Autodesk Inventor part; units mm, degrees
ref_plane "YZ Plane" through (0, 0, 0) normal (1, 0, 0) x (0, 1, 0)
ref_plane "XZ Plane" through (0, 0, 0) normal (0, 1, 0) x (-1, 0, 0)
ref_plane "XY Plane" through (0, 0, 0) normal (0, 0, 1) x (1, 0, 0)
sketch "Sketch1" plane through (0, 0, 0) normal (0, 1, 0) x (-1, 0, 0)
  line L0 (0, 0) -> (25.4, 0)
  line L1 (25.4, 0) -> (25.4, 50.8)
  line L2 (25.4, 50.8) -> (0, 50.8)
  line L3 (0, 50.8) -> (0, 0)
  line L4 (22.86, 48.26) -> (2.54, 48.26)
  line L5 (2.54, 48.26) -> (2.54, 2.54)
  line L6 (2.54, 2.54) -> (22.86, 2.54)
  line L7 (22.86, 2.54) -> (22.86, 48.26)
  dimension "d0" = 50.8
  dimension "d1" = 25.4
  dimension "d2" = 2.54
  dimension "d3" = 2.54
  dimension "d4" = 2.54
  dimension "d5" = 2.54
extrude "Extrusion1" add sketch "Sketch1" along normal blind 762
sketch "Sketch2" plane through (0, 0, 50.8) normal (1, 0, 0) x (0, 0, -1)
  line L0 (0, 0) -> (50.8, 0)
  line L1 (0, 0) -> (0, 762)
  line L2 (50.8, 0) -> (0, 0)
  line L3 (0, 0) -> (0, 25.4)
  line L4 (0, 25.4) -> (50.8, 25.4)
  line L5 (50.8, 25.4) -> (50.8, 0)
  line L6 (48.26, 0) -> (48.26, 762)
  line L7 (2.54, 0) -> (2.54, 762)
  line L8 (48.26, 2.54) -> (2.54, 2.54)
  line L9 (2.54, 2.54) -> (2.54, 22.86)
  line L10 (2.54, 22.86) -> (48.26, 22.86)
  line L11 (48.26, 22.86) -> (48.26, 2.54)
  dimension "d8" = 25.4
  dimension "d9" = 2.54
  dimension "d10" = 2.54
extrude "Extrusion2" add sketch "Sketch2" along normal blind 406.4 contours L1 L4 L7 L0 | L7 L8 L6 L0 | L6 L4 L5 L0 | L4 L6 L10 L7
sketch "Sketch3" plane through (-25.4, 762, 50.8) normal (0, 0, 1) x (1, 0, 0)
  point P0 (25.4, -762)
sketch "Sketch4" plane through (0, 0, 0) normal (0, -1, 0) x (1, 0, 0)
  line L0 (0, 0) -> (406.4, 0)
  line L1 (406.4, 0) -> (431.8, 0)
  line L2 (431.8, 0) -> (431.8, 50.8)
  line L3 (431.8, 50.8) -> (406.4, 50.8)
  line L4 (406.4, 50.8) -> (406.4, 0)
  line L5 (408.94, 48.26) -> (429.26, 48.26)
  line L6 (429.26, 48.26) -> (429.26, 2.54)
  line L7 (429.26, 2.54) -> (408.94, 2.54)
  line L8 (408.94, 2.54) -> (408.94, 48.26)
  dimension "d13" = 25.4
  dimension "d14" = 2.54
  dimension "d15" = 2.54
  dimension "d16" = 2.54
  dimension "d17" = 2.54
extrude "Extrusion3" add sketch "Sketch4" against normal blind 762
sketch "Sketch6" plane through (-25.4, 0, 0) normal (0, 0, -1) x (-1, 0, 0)
  circle A0 centre (-12.7, 12.7) radius 2.5797
  line L0 (0, 0) -> (0, 762)
  line L1 (-457.2, 0) -> (0, 0)
  circle A1 centre (-12.7, 38.1) radius 2.5797
  circle A2 centre (-12.7, 63.5) radius 2.5797
  circle A3 centre (-38.1, 13.2387) radius 2.5797
  circle A4 centre (-63.5, 12.7) radius 2.5797
  circle A5 centre (-12.7, 12.7) radius 2.5797
  line L2 (0, 0) -> (0, 762)
  line L3 (-457.2, 0) -> (0, 0)
  circle A6 centre (-12.7, 38.1) radius 2.5797
  circle A7 centre (-12.7, 63.5) radius 2.5797
  circle A8 centre (-38.1, 13.2387) radius 2.5797
  circle A9 centre (-63.5, 12.7) radius 2.5797
  line L4 (-25.4, 2.54) -> (-431.8, 2.54)
  line L5 (-228.6, 2.54) -> (-228.6, 762)
  circle A10 centre (-444.5, 12.7) radius 2.5797
  circle A11 centre (-444.5, 38.1) radius 2.5797
  circle A12 centre (-419.1, 13.2387) radius 2.5797
  circle A13 centre (-393.7, 12.7) radius 2.5797
  circle A14 centre (-444.5, 63.5) radius 2.5797
  point P0 (-25.4, 0)
  point P1 (-25.4, 0)
  dimension "d22" = 12.7
  dimension "d23" = 12.7
  dimension "d24" = 5.1594
  dimension "d25" = 25.4
  dimension "d26" = 5.1594
  dimension "d27" = 25.4
  dimension "d28" = 5.1594
  dimension "d29" = 25.4
  dimension "d30" = 5.1594
  dimension "d31" = 12.7
  dimension "d32" = 5.1594
  dimension "d33" = 25.4
  dimension "d36" = 12.7
  dimension "d37" = 12.7
  dimension "d38" = 5.1594
  dimension "d39" = 25.4
  dimension "d40" = 5.1594
  dimension "d41" = 25.4
  dimension "d42" = 5.1594
  dimension "d43" = 25.4
  dimension "d44" = 5.1594
  dimension "d45" = 12.7
  dimension "d46" = 5.1594
  dimension "d47" = 25.4
extrude "Extrusion6" cut sketch "Sketch6" against normal blind 736.6
sketch "Sketch8" plane through (-25.4, 0, 50.8) normal (0, 0, 1) x (1, 0, 0)
  line L0 (25.4, 25.4) -> (25.4, 762)
  line L1 (0, 0) -> (25.4, 0)
  line L2 (25.4, 0) -> (25.4, 25.4)
  line L3 (25.4, 25.4) -> (0, 25.4)
  line L4 (0, 25.4) -> (0, 0)
  line L5 (2.54, 2.54) -> (22.86, 2.54)
  line L6 (22.86, 2.54) -> (22.86, 22.86)
  line L7 (22.86, 22.86) -> (2.54, 22.86)
  line L8 (2.54, 22.86) -> (2.54, 2.54)
  line L9 (0, 0) -> (457.2, 0)
  point P0 (25.4, 0)
  dimension "d50" = 25.4
  dimension "d51" = 2.54
  dimension "d52" = 0
  dimension "d53" = 2.54
  dimension "d54" = 2.54
  dimension "d55" = 2.54
extrude "Extrusion7" add sketch "Sketch8" along normal blind 127
sketch "Sketch10" plane through (406.4, 762, 50.8) normal (0, 0, 1) x (1, 0, 0)
  line L0 (0, -736.6) -> (0, 0)
  line L1 (0, -736.6) -> (0, -762)
  point P0 (-406.4, -762)
sketch "Sketch11" plane through (406.4, 762, 50.8) normal (0, 0, 1) x (1, 0, 0)
  line L0 (-406.4, -762) -> (-406.4, -736.6)
  line L1 (-406.4, -762) -> (-406.4, -736.6)
sketch "Sketch12" plane through (406.4, 762, 50.8) normal (0, 0, 1) x (1, 0, 0)
  line L0 (0, -736.6) -> (0, 0)
  line L1 (25.4, -762) -> (25.4, 0)
  line L2 (0, -736.6) -> (25.4, -736.6)
  line L3 (25.4, -736.6) -> (25.4, -762)
  line L4 (25.4, -762) -> (0, -762)
  line L5 (0, -762) -> (0, -736.6)
  line L6 (22.86, -762) -> (22.86, 0)
  line L7 (22.86, -739.14) -> (2.54, -739.14)
  line L8 (2.54, -739.14) -> (2.54, -759.46)
  line L9 (2.54, -759.46) -> (22.86, -759.46)
  line L10 (22.86, -759.46) -> (22.86, -739.14)
  point P0 (-406.4, -762)
  dimension "d62" = 2.54
  dimension "d63" = 2.54
  dimension "d64" = 2.54
extrude "Extrusion9" add sketch "Sketch12" along normal blind 127 contours L4 L6 L2 L1 | L4 L5 L2 L6 L7 L8 L9
sketch "Sketch9" plane through (-25.4, 0, 0) normal (-1, 0, 0) x (0, 0, 1)
  circle A0 centre (64.7925, 12.7) radius 9.525
  line L0 (0, 0) -> (177.8, 0)
  dimension "d58" = 19.05
  dimension "d59" = 12.7
extrude "Extrusion8" cut sketch "Sketch9" against normal blind 508
sketch "Sketch13" plane through (0, 0, 50.8) normal (1, 0, 0) x (0, 0, -1)
  line L0 (-127, 0) -> (-101.6, 0)
  line L1 (-101.6, 0) -> (-101.6, 25.4)
  line L2 (-101.6, 25.4) -> (-127, 25.4)
  line L3 (-127, 25.4) -> (-127, 0)
  line L4 (0, 0) -> (-127, 0)
  line L5 (-127, 0) -> (-127, 25.4)
  line L6 (0, 2.54) -> (-127, 2.54)
  line L7 (-104.14, 2.54) -> (-124.46, 2.54)
  line L8 (-124.46, 2.54) -> (-124.46, 22.86)
  line L9 (-124.46, 22.86) -> (-104.14, 22.86)
  line L10 (-104.14, 22.86) -> (-104.14, 2.54)
  point P0 (50.8, 0)
  dimension "d67" = 25.4
  dimension "d68" = 25.4
  dimension "d69" = 0
  dimension "d70" = 0
  dimension "d71" = 2.54
  dimension "d72" = 2.54
  dimension "d73" = 2.54
extrude "Extrusion10" add sketch "Sketch13" along normal blind 406.4 contours L3 L6 L1 L0 | L3 L2 L1 L6 L10 L9 L8
sketch "Sketch14" plane through (-25.4, 25.4, 50.8) normal (0, 1, 0) x (1, 0, 0)
  line L0 (457.2, -127) -> (0, -127)
  line L1 (228.6, -127) -> (228.6, 50.8)
  line L2 (25.4, 50.8) -> (431.8, 50.8)
  circle A0 centre (444.5, -114.3) radius 2.5797
  circle A1 centre (419.1, -114.3) radius 2.5797
  circle A2 centre (393.7, -114.3) radius 2.5797
  circle A3 centre (444.5, -88.9) radius 2.5797
  circle A4 centre (444.5, -63.5) radius 2.5797
  line L3 (457.2, 0) -> (457.2, -127)
  circle A5 centre (12.7, -114.3) radius 2.5797
  circle A6 centre (38.1, -114.3) radius 2.5797
  circle A7 centre (63.5, -114.3) radius 2.5797
  circle A8 centre (12.7, -88.9) radius 2.5797
  circle A9 centre (12.7, -63.5) radius 2.5797
  dimension "d76" = 90
  dimension "d77" = 228.6
  dimension "d78" = 12.7
  dimension "d79" = 12.7
  dimension "d80" = 12.7
  dimension "d81" = 12.7
  dimension "d82" = 12.7
  dimension "d83" = 12.7
  dimension "d84" = 5.1594
  dimension "d85" = 5.1594
  dimension "d86" = 5.1594
  dimension "d87" = 5.1594
  dimension "d88" = 5.1594
  dimension "d89" = 25.4
  dimension "d90" = 25.4
  dimension "d91" = 25.4
  dimension "d92" = 25.4
extrude "Extrusion11" cut sketch "Sketch14" against normal blind 406.4
properties part number "battery shelf frame"
Could you check a few things on this model? Use its own coordinates, in mm. A direction names the side the tool comes from. Give positions to 0.01 mm unless a question says otherwise; leave off trailing zeros. Order: outer loops, then holes, each group sorted by start corner. A loop starts at its lowest first (then second) coordinate and runs counter-clockwise, first axis right, second up. Notation, with made-up numbers: (60, 26.5) -> (76, 26.5) arc R35 ccw to (76, 65.5) -> close; hole circle Ø1 at (23, 63.25). An arc over 180 degrees is marked (long way). Answer in a Markdown table with one row per item. Add a question column.
Item 1: We'd pull the mould along Y, two halves only. Please class faces 5 (the flat face through (-8, 22.86, 113)), 6 (the flat face through (200, 13, 2.54)), 7 (the flat face through (200, 25.4, 26)), 8 (the flat face through (429.26, 376, 26)): pulls with the +Y half, pulls with the -Y half, needs draft (parallel to the pull), parting line crosses it, or undercut.
Item 2: Imagine slicing it at A-A (x = 126). List the corners of the cut face in (y, z) for me.
Item 3: Please list where these lines run through material, in increasing order: probe 1 along X at (y, z) = (719, 18.5); probe 2 along Z at (x, y) = (419.1, 23.8); probe 3 along Y at (x, z) = (419, 1).
Item 4: For faces 1 (the flat face through (-22.86, 13, 128)), 2 (the flat face through (200, 13, 152.4)), 3 (the flat face through (406.4, 13, 26)), 4 (the flat face through (0, 389, 26)), which set-ups out of +Z, -Z, +X, -X, +Y, -Y let a thin tool reach every point of the face, with its end or its side?
Item 5: Imagine slicing it at C-C (z = 31.5). List the corners of the cut face in (x, y) for me.
Item 6: I'm going to push flat-ended pins straight in: P1, Ø3, axis at x = 419.1, z = 139.7, coming from the -Y side; P2, Ø3, axis at x = 368.3, y = 12.7, coming from the -Z side; P3, Ø6, axis at x = 291.5, z = 49.5, coming from the +Y side. Where does each tip first touch, or does it pass through?
Item 7: Imagine slicing it at B-B (y = 297.5). List the corners of the cut face in (x, z) for me.
Result:
| question | item | result |
|---|---|---|
| 1 | face 5 | undercut |
| 1 | face 6 | undercut |
| 1 | face 7 | pulls with the +Y half |
| 1 | face 8 | needs draft |
| 2 | outline | (0, 0) -> (25.4, 0) -> (25.4, 50.8) -> (0, 50.8) -> close; (0, 152.4) -> (25.4, 152.4) -> (25.4, 177.8) -> (0, 177.8) -> close; hole (2.54, 2.54) -> (22.86, 2.54) -> (22.86, 48.26) -> (2.54, 48.26) -> close; hole (2.54, 154.94) -> (22.86, 154.94) -> (22.86, 175.26) -> (2.54, 175.26) -> close |
| 3 | probe 1 | -25.4 to -22.86, -2.54 to 0, 406.4 to 408.94, 429.26 to 431.8 |
| 3 | probe 2 | 0 to 2.54, 48.26 to 111.72, 116.88 to 137.12, 142.28 to 162.52, 167.68 to 177.8 |
| 3 | probe 3 | 0 to 10.12, 15.28 to 35.52, 40.68 to 60.92, 66.08 to 762 |
| 4 | face 1 | +Z |
| 4 | face 2 | +Y, -Y |
| 4 | face 3 | none |
| 4 | face 4 | +Z, -Z, +Y |
| 5 | outline | (-25.4, 0) -> (-22.86, 0) -> (-22.86, 762) -> (-25.4, 762) -> close; (-2.54, 0) -> (408.94, 0) -> (408.94, 762) -> (406.4, 762) -> (406.4, 25.4) -> (0, 25.4) -> (0, 762) -> (-2.54, 762) -> close; (429.26, 0) -> (431.8, 0) -> (431.8, 762) -> (429.26, 762) -> close; hole (0, 2.54) -> (406.4, 2.54) -> (406.4, 22.86) -> (0, 22.86) -> close |
| 6 | P1 | through |
| 6 | P2 | z = 152.4 |
| 6 | P3 | y = 25.4 |
| 7 | outline | (-25.4, 0) -> (0, 0) -> (0, 50.8) -> (-25.4, 50.8) -> close; (406.4, 0) -> (431.8, 0) -> (431.8, 50.8) -> (406.4, 50.8) -> close; hole (-22.86, 2.54) -> (-2.54, 2.54) -> (-2.54, 48.26) -> (-22.86, 48.26) -> close; hole (408.94, 2.54) -> (429.26, 2.54) -> (429.26, 48.26) -> (408.94, 48.26) -> close |
